Work out the finished part from the listing and answer in its coordinate system (mm). Face numbers are marked on the shaded views. A direction names the side the tool comes from. Round coordinates to 2 decimals unless told otherwise and drop trailing zeros. Loops run counter-clockwise (first coordinate to the right, second up) from the corner with the lowest first, then second, coordinate; pieces in that order, holes last. Notation, with made-up numbers: (23, 26) - (29, 26) arc R31 ccw to (29, 52) - close; hole circle Ø1 at (66, 69.25). An arc over 180 degrees is marked (long way). Return JSON: item names as keys, results as strings.
from build123d import *

# Parameters (mm, degrees)
F0_R        = 39.1254691666
F1_DEPTH    = 124.46
F2_R        = 35.3178604587
F3_DEPTH    = 82.296
F4_S5_R     = 39.1254691666
F4_T6_DEPTH = 57


# Not quite as in the source:
# - a fillet or chamfer that OpenCascade refuses, or shapes differently, is made with other operations: its cross-section is extruded or revolved along the edge and cut away or added
# - a feature of the source that left no trace in its solid (it failed there, or was rolled back) is left out


with BuildPart() as f1:
    # F0 (on Top) → F1 (new body)
    with BuildSketch(Plane.XY):
        Circle(F0_R)
    extrude(amount=F1_DEPTH)

    # F2 (on Top) → F3 (join)
    with BuildSketch(Plane.XY):
        Circle(F2_R)
    extrude(amount=-F3_DEPTH)

    # F4: chamfer of 3.81 on 3 edges, made by hand


with BuildPart() as f4_tool2:
    # F4_s3 → F4_t4 (revolve)
    with BuildSketch(Plane.XZ):
        Polygon((39.1278604587, 0), (35.3178604587, -3.81), (35.3178604587, 0), align=None)
    revolve(axis=Axis((0, 0, 0), (0, 0, 1)))

    # F4_s5 → F4_t6 (intersect, symmetric)
    with BuildSketch(Plane.XY.offset(-1.9)):
        Circle(F4_S5_R)
    extrude(amount=F4_T6_DEPTH, both=True, mode=Mode.INTERSECT)


with BuildPart() as f1_1:
    add(f1.part)

    # F4_t1: union F4_tool2
    add(f4_tool2.part)

    # F4_s7 → F4_t8 (revolve, cut)
    with BuildSketch(Plane.XZ):
        Polygon((35.3178604587, -78.486), (31.5078604587, -82.296), (35.3178604587, -82.296), align=None)
    revolve(axis=Axis((0, 0, -82.296), (0, 0, 1)), mode=Mode.SUBTRACT)


solid = f1_1.part
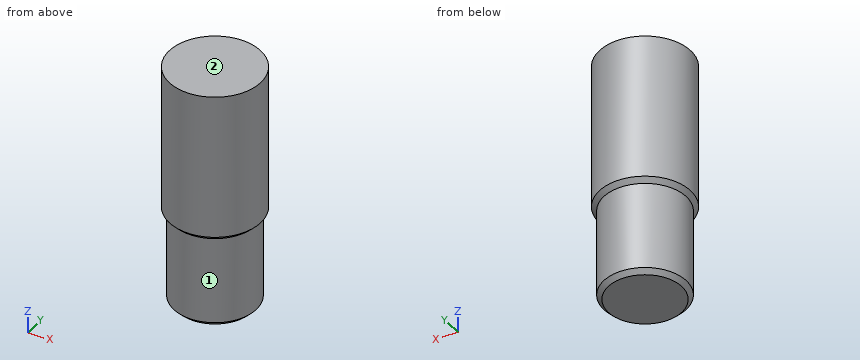
1) A tool of negligible diameter and unlimited length cuts with its end or side. For the marked faces 1 and 2, from which of +Z, -Z, +X, -X, +Y, -Y can it reach the whole face along a straight path? Write none if from no direction.
Verdict:
{"face 1": "-Z", "face 2": "+Z, +X, -X, +Y, -Y"}
2) Find the intervals of material crossed by L1, parallel to Y at x = -18, z = 15.5; L2, parallel to X at y = -8, z = 56.5; L3, parallel to Y at x = -20, z = 50.5, in increasing order.
Verdict:
{"L1": "y = -34.74 to 34.74", "L2": "x = -38.3 to 38.3", "L3": "y = -33.63 to 33.63"}
3) Section A-A (x = 0) is taken. Give the vertices of the cut face in (y, z).
Verdict:
{"outline": "(-39.13, 0) - (-35.32, -3.81) - (-35.32, -78.49) - (-31.51, -82.3) - (31.51, -82.3) - (35.32, -78.49) - (35.32, -3.81) - (39.13, 0) - (39.13, 124.46) - (-39.13, 124.46) - close"}
4) Section C-C (z = 25) is taken. Give the vertices of the cut face in (x, y), and give its area (3 significant figures).
Verdict:
{"outline": "circle Ø78.25 at (0, 0)", "area": "4,810 mm2"}
5) Section D-D (z = -6.5) is taken. Give the vertices of the cut face in (x, y), and give its area (3 significant figures).
Verdict:
{"outline": "circle Ø70.64 at (0, 0)", "area": "3,920 mm2"}
6) Flat-ended cylindrical pins translate along their axes: pin 1 (1.5 mm diameter, centred on y = -20, z = 38.5, fed in from +X); pin 2 (12 mm diameter, centred on x = -12, z = 42.5, fed in from +Y); pin 3 (1.5 mm diameter, centred on x = -3, z = -23.5, fed in from -Y); pin 4 (8 mm diameter, centred on x = -27.5, y = -29.5, fed in from +Z). Find the tip coordinate at first contact, or state that the pin passes through.
Verdict:
{"pin 1": "stops at x = 34.06", "pin 2": "stops at y = 38.66", "pin 3": "stops at y = -35.25", "pin 4": "stops at z = 124.46"}
